Autodesk Inventor part; units mm, degrees
ref_plane "YZ Plane" through (0, 0, 0) normal (1, 0, 0) x (0, 1, 0)
ref_plane "XZ Plane" through (0, 0, 0) normal (0, 1, 0) x (-1, 0, 0)
ref_plane "XY Plane" through (0, 0, 0) normal (0, 0, 1) x (1, 0, 0)
sketch "Sketch1" plane through (0, 0, 0) normal (0, 0, 1) x (1, 0, 0)
  line L0 (0, 0) -> (2400, 0)
  line L1 (2400, 0) -> (2400, 790)
  line L2 (2400, 790) -> (0, 790)
  line L3 (0, 790) -> (0, 0)
  dimension "ancho" = 2400
  dimension "d1" = 790
extrude "Extrusion1" add sketch "Sketch1" along normal blind 50
fillet "Fillet1" radius 50 1 edges at (1200, 0, 50)
sketch "Sketch2" plane through (2400, 790, 50) normal (1, 0, 0) x (0, 0, -1)
  line L0 (50, 0) -> (-50, 0)
  line L1 (-50, 0) -> (-50, 0)
  line L2 (-30, -20) -> (50, -20)
  line L3 (50, -20) -> (50, 0)
  arc A0 (-50, 0) -> (-30, -20) centre (-30, 0) ccw
  point P0 (50, -790)
  point P1 (-50, -20)
  dimension "d5" = 100
  dimension "d6" = 20
  dimension "d7" = 20
extrude "Extrusion2" add sketch "Sketch2" against normal up to surface (2400 mm away)
properties part number "meson"
For this review, take the finished solid that the model builds, in its own axes (mm). A direction names the side the tool comes from. Coordinates: 2 decimals unless noted, no trailing zeros. Loops run counter-clockwise (first coordinate to the right, second up) from the corner with the lowest first, then second, coordinate; pieces in that order, holes last.
1. Add section B-B, the plane y = 491. Give the boundary of the cut face in (x, z), then the cut area to 3 significant figures.
2. For faces 1 (the flat face through (2400, 389, 27)), 2 (the flat face through (1183, 415, 50)), list the 3-axis set-ups (+Z, -Z, +X, -X, +Y, -Y) from which the entire face can be reached by the end or side of a thin tool; tool diameter is ignored.
3. Insertion check: P1, Ø8, axis at x = 1858.5, z = 55.5, coming from the -Y side; P2, Ø2, axis at x = 2061.5, z = 30, coming from the -Y side; P3, Ø1, axis at x = 1416.5, z = 35, coming from the -Y side. Each pin has a flat end and moves straight along its axis. Give the tip position at first contact, or say it passes through.
4. For line 1 (Y direction, x = 1540.5, z = 83); line 2 (Z direction, x = 1098, y = 584.5); line 3 (Y direction, x = 418.5, z = 81), list the stretches that pass through material, from the lowest coordinate up.
Result:
1. outline: (0, 0) - (2400, 0) - (2400, 50) - (0, 50) - close
1. area: 120,000 mm2
2. face 1: +Z, -Z, +X, +Y, -Y
2. face 2: +Z, +X, -X, -Y
3. P1: stops at y = 770
3. P2: stops at y = 9.27
3. P3: stops at y = 13.81
4. line 1: y = 770.23 to 790
4. line 2: z = 0 to 50
4. line 3: y = 770.03 to 790
